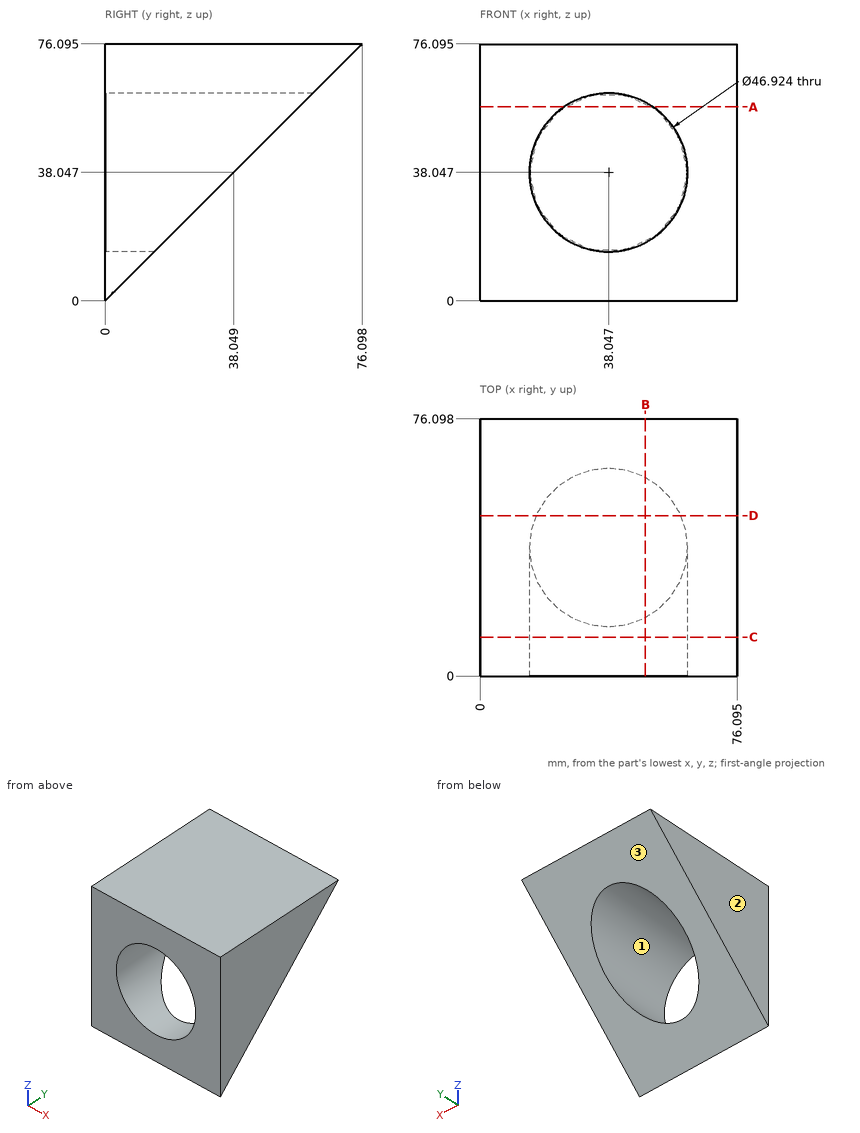
Could you check a few things on this drawing? It's one solid part, dimensions in mm from its lowest x, y, z. Coordinates: 2 decimals unless noted, no trailing zeros. Loops run counter-clockwise (first coordinate to the right, second up) from the corner with the lowest first, then second, coordinate; pieces in that order, holes last. Notation, with made-up numbers: (16, -36) - (60, -36) arc R9 ccw to (60, -24) - close; hole circle Ø6 at (-33, 3). An arc over 180 degrees is marked (long way). Answer as a JSON object with one key per item and string values. Group by question number.
Item 1: For pin 1 (8 mm diameter, centred on x = 40.5, y = 10.5, fed in from -Z); pin 2 (12 mm diameter, centred on x = 27, y = 56.5, fed in from -Z) (1 decimal); pin 3 (10 mm diameter, centred on x = 39.5, y = 40, fed in from -Z) (1 decimal); pin 4 (10 mm diameter, centred on y = 42.5, z = 40, fed in from -X), each with a flat end and sliding along its axis, tell me the tip position at first contact or that it passes through.
Item 2: If we section it at D-D (y = 47.5): List the corners of the cut face in (x, z) for me (1 decimal).
Item 3: If we section it at C-C (y = 11.5): List the corners of the cut face in (x, z) for me (1 decimal), plus the area to 3 significant figures.
Item 4: If we section it at B-B (x = 49): List the corners of the cut face in (y, z) for me (1 decimal), plus the area to 3 significant figures.
Item 5: If I drill on L1, parallel to X at y = 49.5, z = 55 (1 decimal); L2, parallel to X at y = 5, z = 34 (1 decimal); L3, parallel to Y at x = 40.5, z = 10, over which ranges is the centre line in solid material (lowest first)? Write a range as from..to.
Item 6: If we mould it in two halves opening along X, with no side actions, what happens to the marked faces 1, 2 and 3? For each: released by +X, released by -X, zero draft, split by the parting line, or undercut.
Item 7: If we section it at A-A (z = 57.5): List the corners of the cut face in (x, y) for me (1 decimal), plus the area to 3 significant figures.
Returned:
{
 "1": {"pin 1": "stops at z = 6.5", "pin 2": "stops at z = 54.5", "pin 3": "stops at z = 60.6", "pin 4": "stops at x = 0"},
 "2": {"outline": "(0, 47.5) - (16.6, 47.5) arc R23.5 cw to (59.5, 47.5) - (76.1, 47.5) - (76.1, 76.1) - (0, 76.1) - close"},
 "3": {"outline": "(0, 11.5) - (76.1, 11.5) - (76.1, 76.1) - (0, 76.1) - close; hole circle Ø46.9 at (38, 38)", "area": "3,190 mm²"},
 "4": {"outline": "(0, 0) - (17.3, 17.3) - (0, 17.3) - close; (0, 58.8) - (58.8, 58.8) - (76.1, 76.1) - (0, 76.1) - close", "area": "1,320 mm²"},
 "5": {"L1": "x = 0..21.8, 54.3..76.1", "L2": "x = 0..14.9, 61.2..76.1", "L3": "y = 0..10"},
 "6": {"face 1": "undercut", "face 2": "released by -X", "face 3": "zero draft"},
 "7": {"outline": "(0, 0) - (24.9, 0) - (24.9, 57.5) - (0, 57.5) - close; (51.2, 0) - (76.1, 0) - (76.1, 57.5) - (51.2, 57.5) - close", "area": "2,870 mm²"}
}
